Can you work these out from the model? Positions are in its coordinate system, mm. Face numbers are marked on the shaded views. A direction names the side the tool comes from. Give positions to 0.01 mm unless a question says otherwise; leave off trailing zeros. Loops run counter-clockwise (first coordinate to the right, second up) from the corner with the lowest first, then second, coordinate; pieces in that order, holes last. Notation, with made-up numbers: (87.25, -8.75) - (132.25, -8.75) arc R15 cw to (132.25, 18.25) - close; hole circle Ø2 at (-7.75, 86.5). An arc over 180 degrees is marked (long way). Answer in a Markdown table with one row per item.
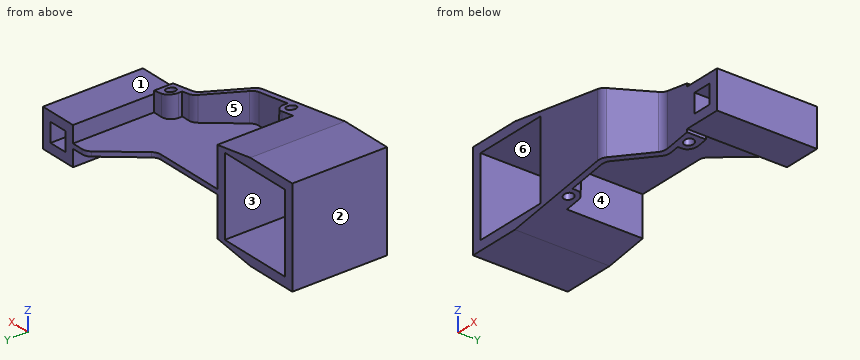
from build123d import *

# Parameters (mm, degrees)
SKETCH1_W           = 275
SKETCH1_H           = 102.5
BOSS_EXTRUDE1_DEPTH = 145.5
SKETCH2_W           = 168
SKETCH2_H           = 102.5
CUT_EXTRUDE1_DEPTH  = 45.5
SKETCH3_W           = 68
SKETCH3_H           = 48.75
CUT_EXTRUDE2_DEPTH  = 80
SKETCH4_W           = 80
SKETCH4_H           = 82.5
CUT_EXTRUDE3_DEPTH  = 311.050399129
SKETCH5_R           = 5
CUT_EXTRUDE4_DEPTH  = 48.75
SKETCH6_R           = 5
CUT_EXTRUDE5_DEPTH  = 48.75
SKETCH5_2_R         = 5
CUT_EXTRUDE6_DEPTH  = 328.569076685
CUT_EXTRUDE7_DEPTH  = 328.569076685
CUT_EXTRUDE8_DEPTH  = 328.569076685
CUT_EXTRUDE9_DEPTH  = 48.75
SKETCH10_R          = 5
CUT_EXTRUDE10_DEPTH = 48.75
SKETCH11_W          = 40
SKETCH11_H          = 31.25
CUT_EXTRUDE11_DEPTH = 328.569076685
SKETCH12_W          = 20
SKETCH12_H          = 20
CUT_EXTRUDE12_DEPTH = 328.569076685
SKETCH13_R          = 5
CUT_EXTRUDE13_DEPTH = 316.728225694
CUT_EXTRUDE14_DEPTH = 311.050399129
FILLET1_R           = 10
FILLET2_R           = 10


with BuildPart() as part:
    # Sketch1 → Boss-Extrude1 (new body)
    with BuildSketch(Plane(origin=(0, 0, 0), x_dir=(1, 0, 0), z_dir=(0, 1, 0))):
        with Locations((-137.5, -51.25)):
            Rectangle(SKETCH1_W, SKETCH1_H)
    extrude(amount=BOSS_EXTRUDE1_DEPTH)

    # Sketch2 → Cut-Extrude1 (cut)
    with BuildSketch(Plane(origin=(0, 145.5, 0), x_dir=(1, 0, 0), z_dir=(0, 1, 0))):
        with Locations((-191, -51.25)):
            Rectangle(SKETCH2_W, SKETCH2_H)
    extrude(amount=-CUT_EXTRUDE1_DEPTH, mode=Mode.SUBTRACT)

    # Sketch3 → Cut-Extrude2 (cut)
    with BuildSketch(Plane(origin=(0, 100, 0), x_dir=(1, 0, 0), z_dir=(0, 1, 0))):
        with Locations((-141, -24.375)):
            Rectangle(SKETCH3_W, SKETCH3_H)
        with Locations((-141, -78.125)):
            Rectangle(SKETCH3_W, SKETCH3_H)
    extrude(amount=-CUT_EXTRUDE2_DEPTH, mode=Mode.SUBTRACT)

    # Sketch4 → Cut-Extrude3 (cut, through all)
    with BuildSketch(Plane(origin=(0, 100, 0), x_dir=(1, 0, 0), z_dir=(0, 1, 0))):
        with Locations((-225, -51.25)):
            Rectangle(SKETCH4_W, SKETCH4_H)
    extrude(amount=-CUT_EXTRUDE3_DEPTH, mode=Mode.SUBTRACT)

    # Sketch5 → Cut-Extrude4 (cut)
    with BuildSketch(Plane.XY.offset(102.5)):
        with Locations((-160, 10)):
            Circle(SKETCH5_R)
        with BuildLine():
            Line((-107, 6), (-150, 6))
            Line((-150, 6), (-150, 10))
            ThreePointArc((-150, 10), (-152.928932188, 17.071067812), (-160, 20))
            Line((-160, 20), (-175, 20))
            Line((-175, 20), (-175, 100))
            Line((-175, 100), (-107, 100))
            Line((-107, 100), (-107, 6))
        make_face()
    extrude(amount=-CUT_EXTRUDE4_DEPTH, mode=Mode.SUBTRACT)

    # Sketch6 → Cut-Extrude5 (cut)
    with BuildSketch(Plane(origin=(0, 0, 0), x_dir=(-1, 0, 0), z_dir=(0, 0, -1))):
        with Locations(Location((160, 10, 0), (0, 0, 180))):
            Circle(SKETCH6_R)
        with BuildLine():
            Line((107, 100), (175, 100))
            Line((175, 100), (175, 20))
            Line((175, 20), (160, 20))
            ThreePointArc((160, 20), (152.928932188, 17.071067812), (150, 10))
            Line((150, 10), (150, 6))
            Line((150, 6), (107, 6))
            Line((107, 6), (107, 100))
        make_face()
    extrude(amount=-CUT_EXTRUDE5_DEPTH, mode=Mode.SUBTRACT)

    # Sketch5_2 → Cut-Extrude6 (cut, through all)
    with BuildSketch(Plane.XY.offset(102.5)):
        with Locations((-160, 10)):
            Circle(SKETCH5_2_R)
    extrude(amount=-CUT_EXTRUDE6_DEPTH, mode=Mode.SUBTRACT)

    # Sketch7 → Cut-Extrude7 (cut, through all)
    with BuildSketch(Plane.XY.offset(102.5)):
        Polygon((0, 40), (-70.638168804, 40), (-104.202154051, 0), (0, 0), align=None)
    extrude(amount=-CUT_EXTRUDE7_DEPTH, mode=Mode.SUBTRACT)

    # Sketch8 → Cut-Extrude8 (cut, through all)
    with BuildSketch(Plane.XY.offset(102.5)):
        Polygon((-107, 145.5), (-107, 100), (-95.026758248, 100), (-56.847725029, 145.5), align=None)
    extrude(amount=-CUT_EXTRUDE8_DEPTH, mode=Mode.SUBTRACT)

    # Sketch9 → Cut-Extrude9 (cut)
    with BuildSketch(Plane.XY.offset(102.5)):
        with BuildLine():
            Line((-40, 145.5), (-40, 60))
            Line((-40, 60), (-50, 60))
            ThreePointArc((-50, 60), (-57.071067812, 57.071067812), (-60, 50))
            Line((-60, 50), (-60, 46))
            Line((-60, 46), (-73.436014753, 46))
            Line((-73.436014753, 46), (-107, 6))
            Line((-107, 6), (-107, 100))
            Line((-107, 100), (-95.026758248, 100))
            Line((-95.026758248, 100), (-56.847725029, 145.5))
            Line((-56.847725029, 145.5), (-40, 145.5))
        make_face()
    extrude(amount=-CUT_EXTRUDE9_DEPTH, mode=Mode.SUBTRACT)

    # Sketch10 → Cut-Extrude10 (cut)
    with BuildSketch(Plane(origin=(0, 0, 0), x_dir=(-1, 0, 0), z_dir=(0, 0, -1))):
        with Locations((50, 50)):
            Circle(SKETCH10_R)
        with BuildLine():
            Line((40, 145.5), (40, 60))
            Line((40, 60), (50, 60))
            ThreePointArc((50, 60), (57.071067812, 57.071067812), (60, 50))
            Line((60, 50), (60, 46))
            Line((60, 46), (73.436014753, 46))
            Line((73.436014753, 46), (107, 6))
            Line((107, 6), (107, 100))
            Line((107, 100), (95.026758248, 100))
            Line((95.026758248, 100), (56.847725029, 145.5))
            Line((56.847725029, 145.5), (40, 145.5))
        make_face()
    extrude(amount=-CUT_EXTRUDE10_DEPTH, mode=Mode.SUBTRACT)

    # Sketch11 → Cut-Extrude11 (cut, through all)
    with BuildSketch(Plane(origin=(0, 145.5, 0), x_dir=(1, 0, 0), z_dir=(0, 1, 0))):
        with Locations((-20, -86.875)):
            Rectangle(SKETCH11_W, SKETCH11_H)
        with Locations((-20, -15.625)):
            Rectangle(SKETCH11_W, SKETCH11_H)
    extrude(amount=-CUT_EXTRUDE11_DEPTH, mode=Mode.SUBTRACT)

    # Sketch12 → Cut-Extrude12 (cut, through all)
    with BuildSketch(Plane(origin=(0, 145.5, 0), x_dir=(1, 0, 0), z_dir=(0, 1, 0))):
        with Locations((-20, -51.25)):
            Rectangle(SKETCH12_W, SKETCH12_H)
    extrude(amount=-CUT_EXTRUDE12_DEPTH, mode=Mode.SUBTRACT)

    # Sketch13 → Cut-Extrude13 (cut, through all)
    with BuildSketch(Plane(origin=(0, 0, 48.75), x_dir=(-1, 0, 0), z_dir=(0, 0, -1))):
        with Locations((50, 50)):
            Circle(SKETCH13_R)
    extrude(amount=-CUT_EXTRUDE13_DEPTH, mode=Mode.SUBTRACT)

    # Sketch14 → Cut-Extrude14 (cut, through all)
    with BuildSketch(Plane(origin=(0, 100, 0), x_dir=(1, 0, 0), z_dir=(0, 1, 0))):
        Polygon((-219, 0), (-20, -31.25), (-20, 0), align=None)
        Polygon((-219, -102.5), (-20, -71.25), (-20, -102.5), align=None)
    extrude(amount=-CUT_EXTRUDE14_DEPTH, mode=Mode.SUBTRACT)

    # Fillet1
    fillet1_edges = [part.edges().sort_by_distance(p)[0] for p in [
        (-107, 6, 33.168969849),
        (-73.436014753, 46, 66.695666988),
        (-56.847725029, 145.5, 51.25),
        (-95.026758248, 100, 51.25),
        (-73.436014753, 46, 35.804333012),
        (-107, 6, 69.331030151),
    ]]
    fillet(fillet1_edges, radius=FILLET1_R)

    # Fillet2
    fillet2_edges = [part.edges().sort_by_distance(p)[0] for p in [
        (-104.202154051, 0, 51.25),
        (-70.638168804, 40, 51.25),
    ]]
    fillet(fillet2_edges, radius=FILLET2_R)


solid = part.part
Q1. Imagine slicing it at A-A, the plane z = 57.5. Count the separate pieces of the cut face and the enclosed holes in it, and give its area (3 significant figures).
Checked values:
| item | result |
|---|---|
| separate pieces | 3 |
| enclosed holes | 2 |
| area | 5,460 mm² |
Q2. Imagine slicing it at B-B, the plane x = -222.5. Write out the boundary of the cut face in (y, z).
Checked values:
| item | result |
|---|---|
| outline | (0, 0) - (100, 0) - (100, 10) - (0, 10) - close; (0, 92.5) - (100, 92.5) - (100, 102.5) - (0, 102.5) - close |
Q3. On a 3-axis mill with a long thin cutter (end or side, diameter ignored), from which of +Z, -Z, +X, -X, +Y, -Y can I reach the whole of each face in a straight line? I mean the marked faces 4, 5 and 6. Say none if no direction works.
Checked values:
| item | result |
|---|---|
| face 4 | -Z, +Y |
| face 5 | +Z, +Y |
| face 6 | +Y, -Y |
Q4. For pin 1 (4.5 mm diameter, centred on y = 7, z = 67, fed in from +X); pin 2 (5 mm diameter, centred on x = -62, z = 44, fed in from -Y); pin 3 (2.5 mm diameter, centred on x = -63.5, z = 36, fed in from +Y), each with a flat end and sliding along its axis, tell me the tip position at first contact or that it passes through.
Checked values:
| item | result |
|---|---|
| pin 1 | stops at x = -96.44 |
| pin 2 | stops at y = 40 |
| pin 3 | stops at y = 46 |
Q5. Imagine slicing it at D-D, the plane y = 136. Write out the boundary of the cut face in (x, z), and give its area (3 significant figures).
Checked values:
| item | result |
|---|---|
| outline | (-64.82, 48.75) - (-40, 48.75) - (-40, 31.25) - (0, 31.25) - (0, 71.25) - (-40, 71.25) - (-40, 53.75) - (-64.82, 53.75) - close; hole (-30, 41.25) - (-10, 41.25) - (-10, 61.25) - (-30, 61.25) - close |
| area | 1,320 mm² |
Q6. If I drill on line 1 (Z direction, x = -22, y = 83.5); line 2 (Y direction, x = -50, z = 53); line 3 (Y direction, x = -160, z = 54.5), over which ranges is the centre line in solid material (lowest first)? Write a range as [from, to].
Checked values:
| item | result |
|---|---|
| line 1 | z = [31.25, 41.25], [61.25, 71.25] |
| line 2 | y = [40, 45], [55, 145.5] |
| line 3 | y = [0, 5], [15, 20] |
Q7. If we mould it in two halves opening along Z, with no side actions, what happens to the marked faces 1, 2 and 3? For each: released by +Z, released by -Z, zero draft, split by the parting line, or undercut.
Checked values:
| item | result |
|---|---|
| face 1 | released by +Z |
| face 2 | zero draft |
| face 3 | undercut |
Q8. Imagine slicing it at C-C, the plane y = 84.5. Write out the boundary of the cut face in (x, z), and give its area (3 significant figures).
Checked values:
| item | result |
|---|---|
| outline | (-275, 0) - (-219, 0) - (-175, 6.91) - (-175, 48.75) - (-40, 48.75) - (-40, 31.25) - (0, 31.25) - (0, 71.25) - (-40, 71.25) - (-40, 53.75) - (-175, 53.75) - (-175, 95.59) - (-219, 102.5) - (-275, 102.5) - close; hole (-265, 10) - (-185, 10) - (-185, 92.5) - (-265, 92.5) - close; hole (-30, 41.25) - (-10, 41.25) - (-10, 61.25) - (-30, 61.25) - close |
| area | 5,220 mm² |
